```python
from build123d import *

# Parameters (mm, degrees)
F0_W     = 44.45
F0_H     = 44.45
F1_DEPTH = 304.8
F2_R     = 5.55625
F3_DEPTH = 50.8
F4_R     = 5.55625
F5_DEPTH = 50.8


with BuildPart() as f1:
    # F0 (on Front) → F1 (new body, symmetric)
    with BuildSketch(Plane.XZ):
        with BuildLine():
            Line((-47.625, 0), (-3.175, 0))
            ThreePointArc((-3.175, 0), (-0.929936, 0.929936), (0, 3.175))
            Line((0, 3.175), (0, 47.625))
            ThreePointArc((0, 47.625), (-0.929936, 49.870064), (-3.175, 50.8))
            Line((-3.175, 50.8), (-47.625, 50.8))
            ThreePointArc((-47.625, 50.8), (-49.870064, 49.870064), (-50.8, 47.625))
            Line((-50.8, 47.625), (-50.8, 3.175))
            ThreePointArc((-50.8, 3.175), (-49.870064, 0.929936), (-47.625, 0))
        make_face()
        with Locations((-25.4, 25.4)):
            Rectangle(F0_W, F0_H, mode=Mode.SUBTRACT)
    extrude(amount=F1_DEPTH, both=True)

    # F2 (on face) → F3 (cut)
    with BuildSketch(Plane(origin=(-50.8, 0, 0), x_dir=(0, -1, 0), z_dir=(-1, 0, 0))):
        with Locations((-292.1, 25.4)):
            Circle(F2_R)
        with Locations((-266.7, 25.4)):
            Circle(F2_R)
        with Locations((-241.3, 25.4)):
            Circle(F2_R)
        with Locations((-215.9, 25.4)):
            Circle(F2_R)
        with Locations((-190.5, 25.4)):
            Circle(F2_R)
        with Locations((-165.1, 25.4)):
            Circle(F2_R)
        with Locations((-139.7, 25.4)):
            Circle(F2_R)
        with Locations((-114.3, 25.4)):
            Circle(F2_R)
        with Locations((-88.9, 25.4)):
            Circle(F2_R)
        with Locations((-63.5, 25.4)):
            Circle(F2_R)
        with Locations((-38.1, 25.4)):
            Circle(F2_R)
        with Locations((-12.7, 25.4)):
            Circle(F2_R)
        with Locations((12.7, 25.4)):
            Circle(F2_R)
        with Locations((38.1, 25.4)):
            Circle(F2_R)
        with Locations((63.5, 25.4)):
            Circle(F2_R)
        with Locations((88.9, 25.4)):
            Circle(F2_R)
        with Locations((114.3, 25.4)):
            Circle(F2_R)
        with Locations((139.7, 25.4)):
            Circle(F2_R)
        with Locations((165.1, 25.4)):
            Circle(F2_R)
        with Locations((190.5, 25.4)):
            Circle(F2_R)
        with Locations((215.9, 25.4)):
            Circle(F2_R)
        with Locations((241.3, 25.4)):
            Circle(F2_R)
        with Locations((266.7, 25.4)):
            Circle(F2_R)
        with Locations((292.1, 25.4)):
            Circle(F2_R)
    extrude(amount=-F3_DEPTH, mode=Mode.SUBTRACT)

    # F4 (on face) → F5 (cut)
    with BuildSketch(Plane.XY.offset(50.8)):
        with Locations((-25.4, -292.1)):
            Circle(F4_R)
        with Locations((-25.4, -266.7)):
            Circle(F4_R)
        with Locations((-25.4, -241.3)):
            Circle(F4_R)
        with Locations((-25.4, -215.9)):
            Circle(F4_R)
        with Locations((-25.4, -190.5)):
            Circle(F4_R)
        with Locations((-25.4, -165.1)):
            Circle(F4_R)
        with Locations((-25.4, -139.7)):
            Circle(F4_R)
        with Locations((-25.4, -114.3)):
            Circle(F4_R)
        with Locations((-25.4, -88.9)):
            Circle(F4_R)
        with Locations((-25.4, -63.5)):
            Circle(F4_R)
        with Locations((-25.4, -38.1)):
            Circle(F4_R)
        with Locations((-25.4, -12.7)):
            Circle(F4_R)
        with Locations((-25.4, 12.7)):
            Circle(F4_R)
        with Locations((-25.4, 38.1)):
            Circle(F4_R)
        with Locations((-25.4, 63.5)):
            Circle(F4_R)
        with Locations((-25.4, 88.9)):
            Circle(F4_R)
        with Locations((-25.4, 114.3)):
            Circle(F4_R)
        with Locations((-25.4, 139.7)):
            Circle(F4_R)
        with Locations((-25.4, 165.1)):
            Circle(F4_R)
        with Locations((-25.4, 190.5)):
            Circle(F4_R)
        with Locations((-25.4, 215.9)):
            Circle(F4_R)
        with Locations((-25.4, 241.3)):
            Circle(F4_R)
        with Locations((-25.4, 266.7)):
            Circle(F4_R)
        with Locations((-25.4, 292.1)):
            Circle(F4_R)
    extrude(amount=-F5_DEPTH, mode=Mode.SUBTRACT)


solid = f1.part
```
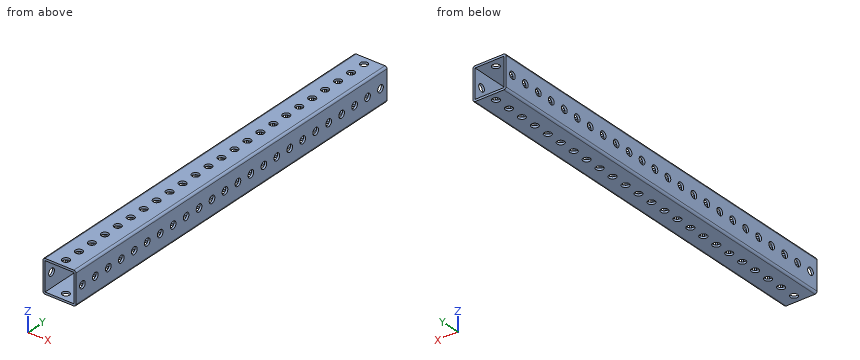
Here's how the part is built. I have some questions about the finished solid (model axes, mm). Round coordinates to 2 decimals unless told otherwise and drop trailing zeros. Order: outer loops, then holes, each group sorted by start corner. A loop starts at its lowest first (then second) coordinate and runs counter-clockwise, first axis right, second up. Notation, with made-up numbers: M 51.5,2 L 76.5,2 A12 cw 76.5,25 Z; hole C 36,25 d10. An arc over 180 degrees is marked long. Answer as CSV lines item,"result".
Item 1: Imagine slicing it at D-D on y = -292.1. List the corners of the cut face in (x, z) for me (3 decimals), and give its area (3 significant figures).
From the geometry:
outline,"M -50.8,3.175 A3.175 ccw -47.625,0 L -30.956,0 L -30.956,3.175 L -47.625,3.175 L -47.625,19.844 L -50.8,19.844 Z; M -50.8,30.956 L -47.625,30.956 L -47.625,47.625 L -30.956,47.625 L -30.956,50.8 L -47.625,50.8 A3.175 ccw -50.8,47.625 Z; M -19.844,0 L -3.175,0 A3.175 ccw 0,3.175 L 0,19.844 L -3.175,19.844 L -3.175,3.175 L -19.844,3.175 Z; M -19.844,47.625 L -3.175,47.625 L -3.175,30.956 L 0,30.956 L 0,47.625 A3.175 ccw -3.175,50.8 L -19.844,50.8 Z"
area,"455 mm2"
Item 2: Imagine slicing it at A-A on z = 38. List the corners of the cut face in (x, y) for me (3 decimals), and give its area (3 significant figures).
From the geometry:
outline,"M -50.8,-304.8 L -47.625,-304.8 L -47.625,304.8 L -50.8,304.8 Z; M -3.175,-304.8 L 0,-304.8 L 0,304.8 L -3.175,304.8 Z"
area,"3,870 mm2"
Item 3: Imagine slicing it at C-C on y = -205. List the corners of the cut face in (x, z) for me (3 decimals).
From the geometry:
outline,"M -50.8,3.175 A3.175 ccw -47.625,0 L -3.175,0 A3.175 ccw 0,3.175 L 0,47.625 A3.175 ccw -3.175,50.8 L -47.625,50.8 A3.175 ccw -50.8,47.625 Z; hole M -47.625,3.175 L -3.175,3.175 L -3.175,47.625 L -47.625,47.625 Z"
Item 4: Imagine slicing it at B-B on x = -39. List the corners of the cut face in (y, z) for me (3 decimals).
From the geometry:
outline,"M -304.8,0 L 304.8,0 L 304.8,3.175 L -304.8,3.175 Z; M -304.8,47.625 L 304.8,47.625 L 304.8,50.8 L -304.8,50.8 Z"
Item 5: Please list where these lines run through material, in increasing order: L1, parallel to Z at x = -43, y = -243 (3 decimals); L2, parallel to X at y = -228, z = 33.5 (3 decimals); L3, parallel to X at y = 241, z = 1. Write a range as [from, to].
From the geometry:
L1,"[0, 3.175], [47.625, 50.8]"
L2,"[-50.8, -47.625], [-3.175, 0]"
L3,"[-49.94, -30.95], [-19.85, -0.86]"
